Part model, mm, in its own coordinate system. Face numbers are marked on the shaded views. A direction names the side the tool comes from. Round coordinates to 2 decimals unless told otherwise and drop trailing zeros. Loops run counter-clockwise (first coordinate to the right, second up) from the corner with the lowest first, then second, coordinate; pieces in that order, holes last. Notation, with made-up numbers: (-35.5, 81.5) -> (-24.5, 81.5) arc R27 ccw to (-24.5, 117.5) -> close; hole circle Ø9 at (-15.75, -6). An arc over 180 degrees is marked (long way). Use a Markdown table: item, result. Add a question column.
Item 1: Cut at A-A, the plane x = 78.5. List the corners of the cut face in (y, z).
Item 2: Two-plate mould, pull along Y, no slides. Class the marked faces 1, 2, 3 and 4: pulls with the +Y half, pulls with the -Y half, needs draft (parallel to the pull), parting line crosses it, or undercut.
Item 3: Cut at D-D, the plane x = 27.5. List the corners of the cut face in (y, z), plus the area to 3 significant figures.
Item 4: Probe line 1 (Y direction, x = 109, z = -57.5); line 2 (Y direction, x = 26.5, z = -58.25); line 3 (Z direction, x = 13, y = 121.5). List the from-to ranges inside material, lowest first. Write a range as [from, to].
Item 5: Cut at C-C, the plane y = 5. List the corners of the cut face in (x, z).
Item 6: Which spindle directions (+Z, -Z, +X, -X, +Y, -Y) get a long thin tool onto all of the face, cutting with end or side? Do the marked faces 5, 6 and 7. Say none if no direction does.
Item 7: Flat gauge pins, fed straight in: pin 1 (12 mm diameter, centred on y = 101, z = -102, fed in from +X); pin 2 (9 mm diameter, centred on x = 40, y = 154, fed in from +Z); pin 3 (6.5 mm diameter, centred on x = 135, y = 23, fed in from -Z); pin 4 (3 mm diameter, centred on x = 135, y = 16, fed in from +Z). Where does each tip first touch, or does it go through?
Item 8: Cut at B-B, the plane y = 166. List the corners of the cut face in (x, z), plus the area to 3 significant figures.
```python
from build123d import *

# Parameters (mm, degrees)
BASE_DEPTH                    = 22.3
RESALTO_FUROS_DE_FIXA_O_DEPTH = 3
SKETCH4_W                     = 105
SKETCH4_H                     = 70
CORPO_RETANGULAR_DEPTH        = 104.2
CORPO_INCLINADO_DEPTH         = 105
SKETCH5_4_R                   = 11.5
CORPO_ARREDONDADO_BACK_DEPTH  = 10
SKETCH5_5_R                   = 11.5
CORPO_ARREDONDADO_FRONT_DEPTH = 125
SKETCH9_R                     = 4
PINOS_GUIA_DEPTH              = 20
RAIOS_50MM_R                  = 50
RAIOS_20MM_R                  = 20
RAIOS_10MM_R                  = 10
RAIOS_5MM_R                   = 5
FURO_M10X50_D                 = 9
FURO_M10X50_DEPTH             = 47.296127214
FURO_M10X50_TIP               = 2.703872786


with BuildPart() as part:
    # Sketch1 → Base (new body)
    with BuildSketch(Plane(origin=(0, 0, 0), x_dir=(1, 0, 0), z_dir=(0, 1, 0))):
        with BuildLine():
            Line((-27.5, 54.25), (-38, 54.25))
            Line((-38, 54.25), (-38, 22.75))
            Line((-38, 22.75), (0, 0))
            Line((0, 0), (104, 0))
            Line((104, 0), (142, 22.75))
            Line((142, 22.75), (142, 54.25))
            Line((142, 54.25), (131.5, 54.25))
            ThreePointArc((131.5, 54.25), (127.5, 58.25), (131.5, 62.25))
            Line((131.5, 62.25), (142, 62.25))
            Line((142, 62.25), (142, 93.75))
            Line((142, 93.75), (104, 116.5))
            Line((104, 116.5), (0, 116.5))
            Line((0, 116.5), (-38, 93.75))
            Line((-38, 93.75), (-38, 62.25))
            Line((-38, 62.25), (-27.5, 62.25))
            ThreePointArc((-27.5, 62.25), (-23.5, 58.25), (-27.5, 54.25))
        make_face()
    extrude(amount=BASE_DEPTH)

    # Sketch3 → Resalto - Furos de Fixa_o (add)
    with BuildSketch(Plane(origin=(0, 22.3, 0), x_dir=(1, 0, 0), z_dir=(0, 1, 0))):
        with BuildLine():
            Line((-27.5, 54.25), (-38, 54.25))
            Line((-38, 54.25), (-38, 48.25))
            Line((-38, 48.25), (-27.5, 48.25))
            ThreePointArc((-27.5, 48.25), (-17.5, 58.25), (-27.5, 68.25))
            Line((-27.5, 68.25), (-38, 68.25))
            Line((-38, 68.25), (-38, 62.25))
            Line((-38, 62.25), (-27.5, 62.25))
            ThreePointArc((-27.5, 62.25), (-23.5, 58.25), (-27.5, 54.25))
        make_face()
        with BuildLine():
            Line((142, 54.25), (142, 48.25))
            Line((142, 48.25), (131.5, 48.25))
            ThreePointArc((131.5, 48.25), (121.5, 58.25), (131.5, 68.25))
            Line((131.5, 68.25), (142, 68.25))
            Line((142, 68.25), (142, 62.25))
            Line((142, 62.25), (131.5, 62.25))
            ThreePointArc((131.5, 62.25), (127.5, 58.25), (131.5, 54.25))
            Line((131.5, 54.25), (142, 54.25))
        make_face()
    extrude(amount=RESALTO_FUROS_DE_FIXA_O_DEPTH)

    # Sketch4 → Corpo Retangular (add)
    with BuildSketch(Plane(origin=(0, 22.3, 0), x_dir=(1, 0, 0), z_dir=(0, 1, 0))):
        with Locations((52, 58.25)):
            Rectangle(SKETCH4_W, SKETCH4_H)
    extrude(amount=CORPO_RETANGULAR_DEPTH)

    # Sketch5 → Corpo Inclinado (add)
    with BuildSketch(Plane.ZY.offset(0.5)):
        Polygon((-58.25, 126.5), (-58.25, 141.5), (-83.25, 141.5), (-93.25, 126.5), align=None)
        Polygon((-33.25, 141.5), (-58.25, 141.5), (-58.25, 126.5), (-23.25, 126.5), align=None)
    extrude(amount=-CORPO_INCLINADO_DEPTH)



with BuildPart() as body_2:
    # Sketch5_4 → Corpo Arredondado - Back (new body)
    with BuildSketch(Plane.ZY.offset(0.5)):
        with BuildLine():
            Line((-33.25, 171.5), (-33.25, 141.5))
            Line((-33.25, 141.5), (-83.25, 141.5))
            Line((-83.25, 141.5), (-83.25, 171.5))
            ThreePointArc((-83.25, 171.5), (-58.25, 196.5), (-33.25, 171.5))
        make_face()
        with Locations((-58.25, 171.5)):
            Circle(SKETCH5_4_R, mode=Mode.SUBTRACT)
    extrude(amount=CORPO_ARREDONDADO_BACK_DEPTH)


with BuildPart() as part_1:
    add(part.part)

    add(body_2.part)  # Corpo Arredondado - Front merges body 2
    # Sketch5_5 → Corpo Arredondado - Front (add)
    with BuildSketch(Plane.ZY.offset(0.5)):
        with BuildLine():
            Line((-33.25, 141.5), (-33.25, 171.5))
            ThreePointArc((-33.25, 171.5), (-58.25, 196.5), (-83.25, 171.5))
            Line((-83.25, 171.5), (-83.25, 141.5))
            Line((-83.25, 141.5), (-33.25, 141.5))
        make_face()
        with Locations((-58.25, 171.5)):
            Circle(SKETCH5_5_R, mode=Mode.SUBTRACT)
    extrude(amount=-CORPO_ARREDONDADO_FRONT_DEPTH)

    # Sketch9 → Pinos Guia (add)
    with BuildSketch(Plane.XZ):
        with Locations(Location((2.5, -58.25, 0), (0, 0, 270))):
            Circle(SKETCH9_R)
        with Locations(Location((101.5, -58.25, 0), (0, 0, 270))):
            Circle(SKETCH9_R)
    extrude(amount=PINOS_GUIA_DEPTH)

    # Raios 50mm
    raios_50mm_edges = [part_1.edges().sort_by_distance(p)[0] for p in [
        (0, 11.15, -116.5),
        (104, 11.15, -116.5),
        (104, 11.15, 0),
        (0, 11.15, 0),
    ]]
    fillet(raios_50mm_edges, radius=RAIOS_50MM_R)

    # Raios 20mm
    raios_20mm_edges = [part_1.edges().sort_by_distance(p)[0] for p in [
        (52, 141.5, -83.25),
        (52, 141.5, -33.25),
        (52, 126.5, -93.25),
        (52, 126.5, -23.25),
    ]]
    fillet(raios_20mm_edges, radius=RAIOS_20MM_R)

    # Raios 10mm
    raios_10mm_edges = [part_1.edges().sort_by_distance(p)[0] for p in [
        (-38, 11.15, -22.75),
        (-38, 11.15, -93.75),
        (142, 11.15, -93.75),
        (142, 11.15, -22.75),
    ]]
    fillet(raios_10mm_edges, radius=RAIOS_10MM_R)

    # Raios 5mm
    raios_5mm_edges = [part_1.edges().sort_by_distance(p)[0] for p in [
        (-22.498390623, 22.3, -103.030568772),
        (52, 22.3, -116.5),
        (52, 22.3, 0),
        (126.498390623, 22.3, -13.469431228),
        (103.500210672, 22.3, -1.807799082),
        (0.499789328, 22.3, -1.807799082),
        (103.500210672, 22.3, -114.692200918),
        (0.499789328, 22.3, -114.692200918),
        (-38, 22.3, -78.165851268),
        (-22.498390623, 22.3, -13.469431228),
        (142, 22.3, -38.334148732),
        (126.498390623, 22.3, -103.030568772),
        (140.699613253, 22.3, -23.48709789),
        (140.699613253, 22.3, -93.01290211),
        (-36.699613253, 22.3, -23.48709789),
        (-36.699613253, 22.3, -93.01290211),
        (-38, 22.3, -38.334148732),
        (142, 22.3, -78.165851268),
    ]]
    fillet(raios_5mm_edges, radius=RAIOS_5MM_R)

    # Furo M10x50
    with Locations(Plane.ZY.offset(0.5)):
        with Locations((-58.25, 121.5)):
            Hole(FURO_M10X50_D / 2, depth=FURO_M10X50_DEPTH)
            with Locations((0, 0, -(FURO_M10X50_DEPTH + FURO_M10X50_TIP / 2))):  # 118° drill point
                Cone(0, FURO_M10X50_D / 2, FURO_M10X50_TIP, mode=Mode.SUBTRACT)


solid = part_1.part
```
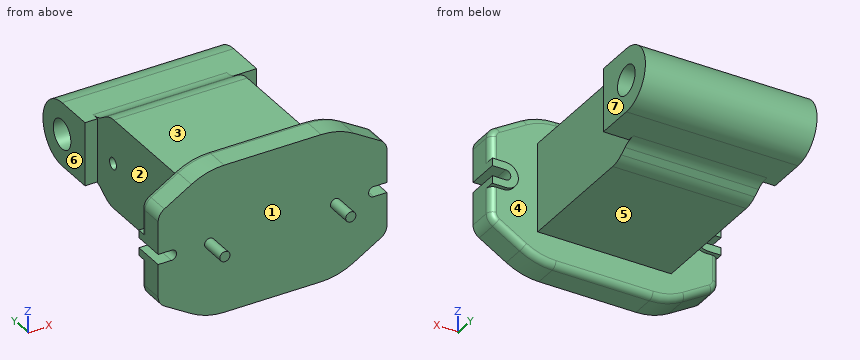
A:
| question | item | result |
|---|---|---|
| 1 | outline | (0, -116.5) -> (17.3, -116.5) arc R5 ccw to (22.3, -111.5) -> (22.3, -93.25) -> (120.44, -93.25) arc R20 ccw to (131.54, -89.89) -> (136.46, -86.61) arc R20 cw to (147.56, -83.25) -> (171.5, -83.25) arc R25 ccw to (171.5, -33.25) -> (147.56, -33.25) arc R20 cw to (136.46, -29.89) -> (131.54, -26.61) arc R20 ccw to (120.44, -23.25) -> (22.3, -23.25) -> (22.3, -5) arc R5 ccw to (17.3, 0) -> (0, 0) -> close; hole circle Ø23 at (171.5, -58.25) |
| 2 | face 1 | pulls with the -Y half |
| 2 | face 2 | undercut |
| 2 | face 3 | needs draft |
| 2 | face 4 | undercut |
| 3 | outline | (0, -116.5) -> (17.3, -116.5) arc R5 ccw to (22.3, -111.5) -> (22.3, -93.25) -> (120.44, -93.25) arc R20 ccw to (131.54, -89.89) -> (136.46, -86.61) arc R20 cw to (147.56, -83.25) -> (171.5, -83.25) arc R25 ccw to (171.5, -33.25) -> (147.56, -33.25) arc R20 cw to (136.46, -29.89) -> (131.54, -26.61) arc R20 ccw to (120.44, -23.25) -> (22.3, -23.25) -> (22.3, -5) arc R5 ccw to (17.3, 0) -> (0, 0) -> close; hole circle Ø9 at (121.5, -58.25); hole circle Ø23 at (171.5, -58.25) |
| 3 | area | 12,800 mm^2 |
| 4 | line 1 | y = [0, 22.3], [141.5, 160.02], [182.98, 196.49] |
| 4 | line 2 | y = [0, 117], [126, 160], [183, 196.5] |
| 4 | line 3 | z = [-93.22, -62.75], [-53.75, -23.28] |
| 5 | outline | (-38, -88.08) arc R10 ccw to (-33.14, -96.66) -> (-11.86, -109.4) arc R50 ccw to (13.82, -116.5) -> (90.18, -116.5) arc R50 ccw to (115.86, -109.4) -> (137.14, -96.66) arc R10 ccw to (142, -88.08) -> (142, -62.25) -> (131.5, -62.25) arc R4 cw to (131.5, -54.25) -> (142, -54.25) -> (142, -28.42) arc R10 ccw to (137.14, -19.84) -> (115.86, -7.1) arc R50 ccw to (90.18, 0) -> (13.82, 0) arc R50 ccw to (-11.86, -7.1) -> (-33.14, -19.84) arc R10 ccw to (-38, -28.42) -> (-38, -54.25) -> (-27.5, -54.25) arc R4 cw to (-27.5, -62.25) -> (-38, -62.25) -> close |
| 6 | face 5 | -Z, +X, -X, +Y |
| 6 | face 6 | +Z, -Z, -X, +Y |
| 6 | face 7 | +Z, -Z, +X, +Y |
| 7 | pin 1 | passes through |
| 7 | pin 2 | stops at z = -33.25 |
| 7 | pin 3 | stops at z = -97.86 |
| 7 | pin 4 | stops at z = -17.66 |
| 8 | outline | (-10.5, -83.25) -> (124.5, -83.25) -> (124.5, -68.35) -> (-10.5, -68.35) -> close; (-10.5, -48.15) -> (124.5, -48.15) -> (124.5, -33.25) -> (-10.5, -33.25) -> close |
| 8 | area | 4,020 mm^2 |
